Check sheet for the modelled part. Datum: model origin and axes. Units: mm. A direction names the side the tool comes from. Give positions to 0.01 mm unless a question says otherwise; leave off trailing zeros. Write each loop counter-clockwise with the first axis right and the second up, starting at its lowest first coordinate (ties: lowest second). Pieces come first, ordered by that corner, then holes. Notation, with made-up numbers: M -26.5,40 L 30.5,40 A23 cw 30.5,49 Z; hole C -38.5,20 d3. An arc over 180 degrees is marked long. Use CSV: the item, a comma, the result in double quotes. Start each with the question number.
1. Cross-section at B-B, the plane z = 0. Enter the section's corners in (x, y).
2. Mould release check, pull along Z, two halves, no side actions. Record for faces 3 (the face through (-0.9, 31.15, -6.87)), 4 (the face through (-1.85, 31.25, 8.35)), 5 (the face through (-8, 31.5, -4)), 6 (the face through (4.38, 14.79, 8.43)): +Z half, -Z half, draft (parallel to the pull), parting line (faces both ways), or undercut.
3. Depth check by flat-ended pin: P1, Ø5, axis at x = 5, y = 22, coming from the -Z side; P2, Ø3, axis at x = 2.5, y = 23, coming from the +Z side; P3, Ø5, axis at x = -3.5, z = -5.5, coming from the -Y side; P4, Ø12, axis at x = 3.5, y = 21.5, coming from the -Z side. Enter the tip coordinate at first touch or a pass-through.
4. Scan lines: line 1 (Z direction, x = 0, y = 31.3); line 2 (Z direction, x = 0, y = 31.15); line 3 (X direction, y = 31.45, z = 0). Record each from-to range of solid material in increasing order.
5. Cross-section at C-C, the plane y = 10.5. Enter the section's corners in (x, z).
6. Access from +Z, -Z, +X, -X, +Y, -Y to the whole of each face (thin tool, end or side, straight path). Record for faces 1 (the face through (-4, 30, -9)), 2 (the face through (0, 31.5, 0)).
7. Cross-section at A-A, the plane x = 0. Enter the section's corners in (y, z).
from build123d import *

# Parameters (mm, degrees)
SKETCH_1_R          = 9.5
EXTRUDE_1_DEPTH     = 30
SKETCH_2_R          = 11.5
EXTRUDE_2_DEPTH     = 1.5
CHAMFER_1_SIZE      = 1
CHAMFER_1_SIZE2     = 2
SKETCH_3_R          = 8.553523617
SKETCH_3_R_2        = 6.929138855
CUT_EXTRUDE_1_DEPTH = 0.5
FILLET_1_R          = 0.2


with BuildPart() as part:
    # 草图1 → 凸台-拉伸1 (new body)
    with BuildSketch(Plane(origin=(0, 0, 0), x_dir=(1, 0, 0), z_dir=(0, 1, 0))):
        Circle(SKETCH_1_R)
    extrude(amount=EXTRUDE_1_DEPTH)

    # 草图2 → 凸台-拉伸2 (add)
    with BuildSketch(Plane(origin=(0, 30, 0), x_dir=(1, 0, 0), z_dir=(0, 1, 0))):
        Circle(SKETCH_2_R)
    extrude(amount=EXTRUDE_2_DEPTH)

    # 倒角1
    chamfer_1_edges = [part.edges().sort_by_distance(p)[0] for p in [
        (-11.5, 31.5, 0),
    ]]
    chamfer_1_side = [part.faces().sort_by_distance(p)[0] for p in [
        (-11.5, 30.75, 0),
    ]]
    chamfer(chamfer_1_edges, length=CHAMFER_1_SIZE, length2=CHAMFER_1_SIZE2, reference=chamfer_1_side[0])

    # 草图3 → 切除-拉伸1 (cut)
    with BuildSketch(Plane(origin=(0, 31.5, 0), x_dir=(1, 0, 0), z_dir=(0, 1, 0))):
        Circle(SKETCH_3_R)
        Circle(SKETCH_3_R_2, mode=Mode.SUBTRACT)
    extrude(amount=-CUT_EXTRUDE_1_DEPTH, mode=Mode.SUBTRACT)

    # 圆角1
    fillet_1_edges = [part.edges().sort_by_distance(p)[0] for p in [
        (-6.929138855, 31.5, 0),
    ]]
    fillet(fillet_1_edges, radius=FILLET_1_R)


solid = part.part
Worked answers:
1,outline,"M -11.5,30 L -9.5,30 L -9.5,0 L 9.5,0 L 9.5,30 L 11.5,30 L 11.5,30.5 L 9.5,31.5 L 8.55,31.5 L 8.55,31 L 6.93,31 L 6.93,31.3 A0.2 ccw 6.73,31.5 L -6.73,31.5 A0.2 ccw -6.93,31.3 L -6.93,31 L -8.55,31 L -8.55,31.5 L -9.5,31.5 L -11.5,30.5 Z"
2,face 3,"undercut"
2,face 4,"undercut"
2,face 5,"draft"
2,face 6,"parting line"
3,P1,"stops at z = -9.17"
3,P2,"stops at z = 9.45"
3,P3,"stops at y = 0"
3,P4,"stops at z = -9.5"
4,line 1,"z = -9.9 to -8.55, -6.93 to 6.93, 8.55 to 9.9"
4,line 2,"z = -10.2 to -8.55, -6.93 to 6.93, 8.55 to 10.2"
4,line 3,"x = -9.6 to -8.55, -6.86 to 6.86, 8.55 to 9.6"
5,outline,"C 0,0 d19"
6,face 1,"-Y"
6,face 2,"+Z, -Z, +X, -X, +Y"
7,outline,"M 0,-9.5 L 30,-9.5 L 30,-11.5 L 30.5,-11.5 L 31.5,-9.5 L 31.5,-8.55 L 31,-8.55 L 31,-6.93 L 31.3,-6.93 A0.2 ccw 31.5,-6.73 L 31.5,6.73 A0.2 ccw 31.3,6.93 L 31,6.93 L 31,8.55 L 31.5,8.55 L 31.5,9.5 L 30.5,11.5 L 30,11.5 L 30,9.5 L 0,9.5 Z"
